from build123d import *

# Parameters (mm, degrees)
SALIENTE_EXTRUIR1_DEPTH  = 111
CROQUIS2_W               = 111
CROQUIS2_H               = 6.192779451
SALIENTE_EXTRUIR2_DEPTH  = 10
CROQUIS3_W               = 111
CROQUIS3_H               = 2.409514801
SALIENTE_EXTRUIR3_DEPTH  = 10
CROQUIS4_W               = 111
CROQUIS4_H               = 2.398640609
SALIENTE_EXTRUIR4_DEPTH  = 10
CROQUIS5_W               = 111
CROQUIS5_H               = 6.192779451
SALIENTE_EXTRUIR5_DEPTH  = 10
CROQUIS6_W               = 111
CROQUIS6_H               = 5
SALIENTE_EXTRUIR6_DEPTH  = 4.321315
CROQUIS7_W               = 111
CROQUIS7_H               = 5
SALIENTE_EXTRUIR7_DEPTH  = 4.278447
CROQUIS8_W               = 111
CROQUIS8_H               = 9
SALIENTE_EXTRUIR8_DEPTH  = 55
CROQUIS9_R               = 2
CORTAR_EXTRUIR1_DEPTH    = 16
CROQUIS10_R              = 4
CORTAR_EXTRUIR2_DEPTH    = 4
CROQUIS11_R              = 2
CORTAR_EXTRUIR3_DEPTH    = 15
CROQUIS12_R              = 4
CORTAR_EXTRUIR4_DEPTH    = 4
SALIENTE_EXTRUIR9_DEPTH  = 5
SALIENTE_EXTRUIR11_DEPTH = 5
CHAFL_N1_SIZE            = 2
CROQUIS17_W              = 111
CROQUIS17_H              = 2.5
CORTAR_EXTRUIR5_DEPTH    = 1
CROQUIS18_W              = 111
CROQUIS18_H              = 2.5
CORTAR_EXTRUIR6_DEPTH    = 1
SALIENTE_EXTRUIR13_DEPTH = 111
CORTAR_EXTRUIR7_DEPTH    = 111


with BuildPart() as part:
    # Croquis1 → Saliente-Extruir1 (new body)
    with BuildSketch(Plane(origin=(0, 0, 0), x_dir=(0, 0, -1), z_dir=(1, 0, 0))):
        with BuildLine():
            Line((7.281662572, 0.608509867), (5.132212893, 1.885171952))
            Line((5.132212893, 1.885171952), (2.982763214, 3.161834037))
            Line((2.982763214, 3.161834037), (5.189506733, 6.877213544))
            Line((5.189506733, 6.877213544), (2.867848216, 7.521933103))
            ThreePointArc((2.867848216, 7.521933103), (2.490196159, 6.4721221), (1.960989109, 5.489948939))
            Line((1.960989109, 5.489948939), (-4.770871258, -1.63199293))
            ThreePointArc((-4.770871258, -1.63199293), (-5.721710129, -2.215627798), (-6.748607586, -2.651753735))
            Line((-6.748607586, -2.651753735), (-5.938704572, -4.909525619))
            Line((-5.938704572, -4.909525619), (-2.388950365, -2.52114656))
            Line((-2.388950365, -2.52114656), (-0.993362777, -4.595353706))
            Line((-0.993362777, -4.595353706), (0.402224811, -6.669560852))
            Line((0.402224811, -6.669560852), (-4.197240467, -9.7642164))
            Line((-4.197240467, -9.7642164), (-4.309282935, -9.839601868))
            Line((-4.309282935, -9.839601868), (-2.319133534, -15.703885515))
            ThreePointArc((-2.319133534, -15.703885515), (1.153217714, -13.714536347), (4.172917336, -11.088484655))
            Line((4.172917336, -11.088484655), (11.905759692, -2.907558323))
            ThreePointArc((11.905759692, -2.907558323), (14.35773408, 0.255123277), (16.14854429, 3.83391247))
            Line((16.14854429, 3.83391247), (10.181567392, 5.490929075))
            Line((10.181567392, 5.490929075), (7.281662572, 0.608509867))
        make_face()
    extrude(amount=SALIENTE_EXTRUIR1_DEPTH)

    # Croquis2 → Saliente-Extruir2 (add)
    with BuildSketch(Plane(origin=(0, 7.722777916, -2.144598757), x_dir=(1, 0, 0), z_dir=(0, 0.963537769, -0.267572359))):
        with Locations((55.5, 11.437493615)):
            Rectangle(CROQUIS2_W, CROQUIS2_H)
    extrude(amount=SALIENTE_EXTRUIR2_DEPTH)

    # Croquis3 → Saliente-Extruir3 (add)
    with BuildSketch(Plane(origin=(0, 7.722777916, -2.144598757), x_dir=(1, 0, 0), z_dir=(0, 0.963537769, -0.267572359))):
        with Locations((55.5, 1.955376092)):
            Rectangle(CROQUIS3_W, CROQUIS3_H)
    extrude(amount=SALIENTE_EXTRUIR3_DEPTH)

    # Croquis4 → Saliente-Extruir4 (add)
    with BuildSketch(Plane(origin=(0, -0.571048753, 7.494993546), x_dir=(1, 0, 0), z_dir=(0, 0.337650839, -0.941271433))):
        with Locations((55.5, 3.409846311)):
            Rectangle(CROQUIS4_W, CROQUIS4_H)
    extrude(amount=-SALIENTE_EXTRUIR4_DEPTH)

    # Croquis5 → Saliente-Extruir5 (add)
    with BuildSketch(Plane(origin=(0, -0.440143301, 7.499157089), x_dir=(1, 0, 0), z_dir=(0, 0.321366103, -0.946955029))):
        with Locations((55.5, 13.022371717)):
            Rectangle(CROQUIS5_W, CROQUIS5_H)
    extrude(amount=-SALIENTE_EXTRUIR5_DEPTH)

    # Croquis6 → Saliente-Extruir6 (add)
    with BuildSketch(Plane(origin=(0, 3.646905534, -2.166073516), x_dir=(1, 0, 0), z_dir=(0, 0.859779871, -0.510664834))):
        with Locations((55.5, 3.44988232)):
            Rectangle(CROQUIS6_W, CROQUIS6_H)
    extrude(amount=SALIENTE_EXTRUIR6_DEPTH)

    # Croquis7 → Saliente-Extruir7 (add)
    with BuildSketch(Plane(origin=(0, 6.51296949, 8.467369412), x_dir=(1, 0, 0), z_dir=(0, 0.558235035, -0.829682858))):
        with Locations((55.5, 13.388637699)):
            Rectangle(CROQUIS7_W, CROQUIS7_H)
    extrude(amount=-SALIENTE_EXTRUIR7_DEPTH)

    # Croquis8 → Saliente-Extruir8 (add)
    with BuildSketch(Plane(origin=(0, 1.611575356, 1.704959012), x_dir=(1, 0, 0), z_dir=(0, 0.686924527, 0.726728762))):
        with Locations((55.5, 0.436755314)):
            Rectangle(CROQUIS8_W, CROQUIS8_H)
    extrude(amount=SALIENTE_EXTRUIR8_DEPTH)

    # Croquis9 → Cortar-Extruir1 (cut)
    with BuildSketch(Plane(origin=(0, -3.888865446, -14.003945532), x_dir=(-1, 0, 0), z_dir=(0, -0.267572359, -0.963537769))):
        with Locations((-86.75, 13.015023554)):
            Circle(CROQUIS9_R)
        with Locations((-55.5, 13.015023554)):
            Circle(CROQUIS9_R)
        with Locations((-24.25, 13.015023554)):
            Circle(CROQUIS9_R)
    extrude(amount=-CORTAR_EXTRUIR1_DEPTH, mode=Mode.SUBTRACT)

    # Croquis10 → Cortar-Extruir2 (cut)
    with BuildSketch(Plane(origin=(0, -3.888865446, -14.003945532), x_dir=(-1, 0, 0), z_dir=(0, -0.267572359, -0.963537769))):
        with Locations((-86.75, 13.015023554)):
            Circle(CROQUIS10_R)
        with Locations((-55.5, 13.015023554)):
            Circle(CROQUIS10_R)
        with Locations((-24.25, 13.015023554)):
            Circle(CROQUIS10_R)
    extrude(amount=-CORTAR_EXTRUIR2_DEPTH, mode=Mode.SUBTRACT)

    # Croquis11 → Cortar-Extruir3 (cut)
    with BuildSketch(Plane(origin=(0, -13.376291354, -4.539483394), x_dir=(1, 0, 0), z_dir=(0, -0.946955029, -0.321366103))):
        with Locations((55.5, 12.242811659)):
            Circle(CROQUIS11_R)
        with Locations((24.25, 12.242811659)):
            Circle(CROQUIS11_R)
        with Locations((86.75, 12.242811659)):
            Circle(CROQUIS11_R)
    extrude(amount=-CORTAR_EXTRUIR3_DEPTH, mode=Mode.SUBTRACT)

    # Croquis12 → Cortar-Extruir4 (cut)
    with BuildSketch(Plane(origin=(0, -13.376291354, -4.539483394), x_dir=(-1, 0, 0), z_dir=(0, -0.946955029, -0.321366103))):
        with Locations((-24.25, -12.242811659)):
            Circle(CROQUIS12_R)
        with Locations((-55.5, -12.242811659)):
            Circle(CROQUIS12_R)
        with Locations((-86.75, -12.242811659)):
            Circle(CROQUIS12_R)
    extrude(amount=-CORTAR_EXTRUIR4_DEPTH, mode=Mode.SUBTRACT)

    # Croquis13 → Saliente-Extruir9 (add)
    with BuildSketch(Plane.ZY):
        with BuildLine():
            Line((-9.48840609, 4.323889374), (3.147529397, -9.057939911))
            Line((3.147529397, -9.057939911), (4.309282935, -9.839601868))
            Line((4.309282935, -9.839601868), (13.778833228, -13.053262902))
            Line((13.778833228, -13.053262902), (11.788683827, -18.917546549))
            Line((11.788683827, -18.917546549), (2.319133534, -15.703885515))
            ThreePointArc((2.319133534, -15.703885515), (-1.153217714, -13.714536347), (-4.172917336, -11.088484655))
            Line((-4.172917336, -11.088484655), (-11.905759692, -2.907558323))
            ThreePointArc((-11.905759692, -2.907558323), (-14.35773408, 0.255123277), (-16.14854429, 3.83391247))
            Line((-16.14854429, 3.83391247), (-18.824267877, 13.469290163))
            Line((-18.824267877, 13.469290163), (-12.857290979, 15.126306768))
            Line((-12.857290979, 15.126306768), (-10.181567392, 5.490929075))
            Line((-10.181567392, 5.490929075), (-9.48840609, 4.323889374))
        make_face()
    extrude(amount=SALIENTE_EXTRUIR9_DEPTH)

    # Croquis15 → Saliente-Extruir11 (add)
    with BuildSketch(Plane(origin=(111, 0, 0), x_dir=(0, 0, -1), z_dir=(1, 0, 0))):
        with BuildLine():
            Line((-3.147529397, -9.057939911), (9.48840609, 4.323889374))
            Line((9.48840609, 4.323889374), (10.181567392, 5.490929075))
            Line((10.181567392, 5.490929075), (12.857290979, 15.126306768))
            Line((12.857290979, 15.126306768), (18.824267877, 13.469290163))
            Line((18.824267877, 13.469290163), (16.14854429, 3.83391247))
            ThreePointArc((16.14854429, 3.83391247), (14.35773408, 0.255123277), (11.905759692, -2.907558323))
            Line((11.905759692, -2.907558323), (4.172917336, -11.088484655))
            ThreePointArc((4.172917336, -11.088484655), (1.153217714, -13.714536347), (-2.319133534, -15.703885515))
            Line((-2.319133534, -15.703885515), (-11.788683827, -18.917546549))
            Line((-11.788683827, -18.917546549), (-13.778833228, -13.053262902))
            Line((-13.778833228, -13.053262902), (-4.309282935, -9.839601868))
            Line((-4.309282935, -9.839601868), (-3.147529397, -9.057939911))
        make_face()
    extrude(amount=SALIENTE_EXTRUIR11_DEPTH)

    # Chaflán1
    chafl_n1_edges = [part.edges().sort_by_distance(p)[0] for p in [
        (55.5, 42.980106436, 38.283862622),
        (55.5, 36.439547576, 44.466183368),
    ]]
    chamfer(chafl_n1_edges, length=CHAFL_N1_SIZE)

    # Croquis17 → Cortar-Extruir5 (cut)
    with BuildSketch(Plane(origin=(0, 3.587682079, -3.391178311), x_dir=(1, 0, 0), z_dir=(0, 0.726728762, -0.686924527))):
        with Locations((55.5, -54.596073392)):
            Rectangle(CROQUIS17_W, CROQUIS17_H)
    extrude(amount=-CORTAR_EXTRUIR5_DEPTH, mode=Mode.SUBTRACT)

    # Croquis18 → Cortar-Extruir6 (cut)
    with BuildSketch(Plane(origin=(0, -2.952876781, 2.791142435), x_dir=(-1, 0, 0), z_dir=(0, -0.726728762, 0.686924527))):
        with Locations((-55.5, -54.596073392)):
            Rectangle(CROQUIS18_W, CROQUIS18_H)
    extrude(amount=-CORTAR_EXTRUIR6_DEPTH, mode=Mode.SUBTRACT)

    # Croquis19 → Saliente-Extruir13 (add)
    with BuildSketch(Plane.ZY):
        Polygon((37.537231743, 41.586355264), (33.072222315, 46.310092218), (22.171290882, 36.006224308), (36.596705955, 20.744920302), (47.497637388, 31.048788212), (43.032627961, 35.772525166), (43.092334313, 37.8930051), (39.657711677, 41.526648911), align=None)
    extrude(amount=-SALIENTE_EXTRUIR13_DEPTH)

    # Croquis20 → Cortar-Extruir7 (cut)
    with BuildSketch(Plane.ZY):
        Polygon((45.713483262, 32.936326171), (39.269105528, 34.936320207), (37.48465455, 30.110641878), (44.275491662, 28.003125173), (47.497637388, 31.048788212), align=None)
        Polygon((33.072222315, 46.310092218), (34.856376442, 44.422554259), (36.490580545, 37.875848411), (31.572137947, 36.36576264), (29.850076589, 43.264429179), align=None)
    extrude(amount=-CORTAR_EXTRUIR7_DEPTH, mode=Mode.SUBTRACT)


solid = part.part
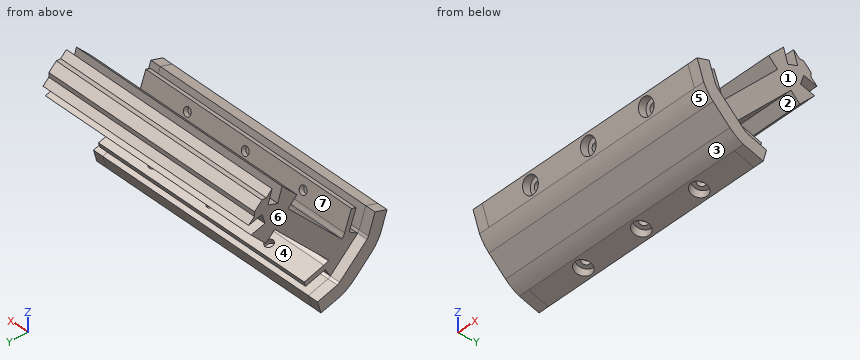
Input: part model. Units: mm. Frame: model coordinates. Face numbers are marked on the shaded views. A direction names the side the tool comes from. Give positions to 0.01 mm unless a question says otherwise; leave off trailing zeros. Loops run counter-clockwise (first coordinate to the right, second up) from the corner with the lowest first, then second, coordinate; pieces in that order, holes last. Notation, with made-up numbers: (82.25, 27.25) -> (104.25, 27.25) arc R17 cw to (104.25, 43.25) -> close; hole circle Ø3 at (-20, 89). An arc over 180 degrees is marked (long way). Answer as a JSON object with one key per item and string values. Group by question number.
Item 1: Pull-direction query (Y, two-part tool) for the marked faces 5, 6 and 7; classes: released by +Y, released by -Y, zero draft, split by the parting line, or undercut.
Item 2: Line query: probe 1 along Y at (x, z) = (23, 5.5); probe 2 along X at (y, z) = (3, 0); probe 3 along Z at (x, y) = (81, 13). Output: solid intervals per line, ascending.
Item 3: Reachability of the marked faces 1, 2, 3 and 4 from +Z, -Z, +X, -X, +Y, -Y: full face, straight path, thin tool, end or side. Return the list, or none.
Item 4: Cut plane A-A, the plane z = 18. Return the cut outline in (x, y).
Item 5: Pin query (flat end, axial travel): P1, Ø4, axis at x = 51.5, y = 18, coming from the -Z side; P2, Ø8, axis at x = 80, y = -2.5, coming from the +Z side; P3, Ø12, axis at y = 13, z = 18, coming from the -X side. Return the tip coordinate at first contact, or that it passes through.
Checks:
{
 "1": {"face 5": "released by -Y", "face 6": "zero draft", "face 7": "undercut"},
 "2": {"probe 1": "y = -12.56 to -10.24, -5.56 to -2.1, -0.39 to 11.99", "probe 2": "x = 0 to 111", "probe 3": "z = -18.69 to -12.27, -6.89 to -4.39, 6.57 to 19.67"},
 "3": {"face 1": "+Z, +X, +Y", "face 2": "-Z, +X, -X", "face 3": "-Z, +X, -X, -Y", "face 4": "+X, -X, +Y"},
 "4": {"outline": "(0, 11.42) -> (111, 11.42) -> (111, 23.81) -> (0, 23.81) -> close"},
 "5": {"P1": "stops at z = -7.87", "P2": "stops at z = 16.16", "P3": "stops at x = 0"}
}
